Could you check a few things on this model? Use its own coordinates, in mm. Give positions to 0.01 mm unless a question says otherwise; leave off trailing zeros. Loops run counter-clockwise (first coordinate to the right, second up) from the corner with the lowest first, then second, coordinate; pieces in that order, holes last. Notation, with made-up numbers: (76, 57.5) -> (129, 57.5) arc R17 ccw to (129, 63.5) -> close; hole circle Ø2 at (87.25, 49). An arc over 180 degrees is marked (long way). Write each question's results on one line, items separated by ' | '. Start each with the question number.
Q1. If we section it at D-D, the plane x = -46: List the corners of the cut face in (y, z) for me.
Q2. Will these pins go through, and if not, where does the flat tip stop? P1, Ø2, axis at y = 2, z = -66, coming from the +X side; P2, Ø1.2, axis at x = -13.5, y = 3, coming from the +Z side; P3, Ø1, axis at y = 4.5, z = -125, coming from the -X side.
Q3. If I drill on line 1 along Z through (x, y) = (2.5, 1.25); line 2 along Z through (x, y) = (-41, 1.5); line 3 along X through (y, z) = (0.75, -17.5), over which ranges is the centre line in solid material (lowest first)?
Q4. If we section it at C-C, the plane z = -110.5: List the corners of the cut face in (x, y) for me, plus the area to 3 significant figures.
Q5. If we section it at A-A, the plane x = -60: List the corners of the cut face in (y, z) for me, plus the area to 3 significant figures.
Q6. If we section it at B-B, the plane y = 5: Give the number of separate pieces and of enclosed holes in the cut face, plus the area to 3 significant figures.
Autodesk Inventor part; units mm, degrees
ref_plane "YZ Plane" through (0, 0, 0) normal (1, 0, 0) x (0, 1, 0)
ref_plane "XZ Plane" through (0, 0, 0) normal (0, 1, 0) x (-1, 0, 0)
ref_plane "XY Plane" through (0, 0, 0) normal (0, 0, 1) x (1, 0, 0)
sketch "Sketch1" plane through (0, 0, 0) normal (0, 1, 0) x (-1, 0, 0)
  line L0 (8, 0) -> (76.1537, -12.0173)
  line L1 (76.1537, -12.0173) -> (76.1537, -54.5039)
  line L2 (76.1537, -54.5039) -> (9.2866, -150)
  line L3 (0, -150) -> (0, 0)
  line L4 (75.1537, -50.7018) -> (69.8292, -46.9735) construction
  line L5 (69.8292, -46.9735) -> (1, -145.2718) construction
  line L6 (1, -145.2718) -> (6.3245, -149) construction
  line L7 (6.3245, -149) -> (75.1537, -50.7018) construction
  line L8 (75.1537, -14.8873) -> (74.0249, -21.2885) construction
  line L9 (74.0249, -21.2885) -> (1, -8.4123) construction
  line L10 (1, -8.4123) -> (2.1287, -2.011) construction
  line L11 (2.1287, -2.011) -> (75.1537, -14.8873) construction
  line L12 (73.1537, -45.9735) -> (66.6537, -45.9735) construction
  line L13 (66.6537, -45.9735) -> (66.6537, -22.2885) construction
  line L14 (66.6537, -22.2885) -> (73.1537, -22.2885) construction
  line L15 (73.1537, -22.2885) -> (73.1537, -45.9735) construction
  line L16 (0, -150) -> (9.2866, -150)
  line L17 (0, 0) -> (8, 0)
  line L18 (66.6537, -51.5086) -> (66.6537, -19.9888)
  point P0 (0, 0)
  dimension "d0" = 6.5
  dimension "d1" = 3
  dimension "d2" = 3
  dimension "d3" = 3
  dimension "d4" = 120
  dimension "d5" = 80
  dimension "d6" = 35
  dimension "d7" = 1
  dimension "d8" = 1
  dimension "d9" = 1
  dimension "d10" = 1
  dimension "d12" = 1
  dimension "d13" = 8
  dimension "d14" = 150
extrude "Extrusion1" add sketch "Sketch1" along normal blind 6.5
chamfer "Chamfer1" distance 2 angle 45 3 edges at (-76.1537, 3.25, -54.5039) (-76.1537, 3.25, -12.0173) (-9.2866, 3.25, -150)
sketch "Sketch3" plane through (0, 6.5, 0) normal (0, 1, 0) x (1, 0, 0)
  line L0 (-10.4338, 148.3617) -> (-75.0065, 56.1423)
  line L1 (-76.1537, 52.5039) -> (-76.1537, 14.0173)
  line L2 (-74.184, 11.67) -> (-8, 0)
  line L3 (0, 0) -> (0, 150)
  line L4 (0, 150) -> (-7.2866, 150)
  line L5 (-6.3245, 149) -> (-1, 145.2718) construction
  line L6 (-1, 145.2718) -> (-69.8292, 46.9735) construction
  line L7 (-69.8292, 46.9735) -> (-75.1537, 50.7018) construction
  line L8 (-75.1537, 50.7018) -> (-6.3245, 149) construction
  line L9 (-73.1537, 45.9735) -> (-66.6537, 45.9735) construction
  line L10 (-66.6537, 45.9735) -> (-66.6537, 22.2885) construction
  line L11 (-66.6537, 22.2885) -> (-73.1537, 22.2885) construction
  line L12 (-73.1537, 22.2885) -> (-73.1537, 45.9735) construction
  line L13 (-74.0249, 21.2885) -> (-75.1537, 14.8873) construction
  line L14 (-75.1537, 14.8873) -> (-2.1287, 2.011) construction
  line L15 (-2.1287, 2.011) -> (-1, 8.4123) construction
  line L16 (-1, 8.4123) -> (-74.0249, 21.2885) construction
  circle A0 centre (-69.9037, 34.131) radius 2.25
  line L17 (-56.0633, 66.6332) -> (-51.4747, 73.1864)
  line L18 (-51.4747, 73.1864) -> (-56.7992, 76.9146)
  line L19 (-56.7992, 76.9146) -> (-61.3878, 70.3614)
  line L20 (-61.3878, 70.3614) -> (-56.0633, 66.6332)
  line L21 (-37.7089, 92.846) -> (-33.1203, 99.3992)
  line L22 (-33.1203, 99.3992) -> (-38.4448, 103.1275)
  line L23 (-38.4448, 103.1275) -> (-43.0334, 96.5743)
  line L24 (-43.0334, 96.5743) -> (-37.7089, 92.846)
  line L25 (-19.3544, 119.0589) -> (-14.7658, 125.6121)
  line L26 (-14.7658, 125.6121) -> (-20.0903, 129.3404)
  line L27 (-20.0903, 129.3404) -> (-24.6789, 122.7871)
  line L28 (-24.6789, 122.7871) -> (-19.3544, 119.0589)
  line L29 (-72.4914, 48.8376) -> (-58.7256, 68.4973) construction
  line L30 (-54.137, 75.0505) -> (-40.3711, 94.7101) construction
  line L31 (-35.7825, 101.2634) -> (-22.0167, 120.923) construction
  line L32 (-17.4281, 127.4762) -> (-3.6622, 147.1359) construction
  line L33 (-16.3, 112.5) -> (-16.3, 108)
  line L34 (0, 108) -> (0, 112.5)
  line L35 (-12.3, 115) -> (-5, 115)
  line L36 (-5, 105.5) -> (-12.3, 105.5)
  line L37 (0, 112.5) -> (-5, 112.5)
  line L38 (-12.3, 112.5) -> (-16.3, 112.5)
  line L39 (-16.3, 108) -> (-12.3, 108)
  line L40 (-5, 108) -> (0, 108)
  line L41 (-12.3, 105.5) -> (-12.3, 108)
  line L42 (-12.3, 112.5) -> (-12.3, 115)
  line L43 (-5, 115) -> (-5, 112.5)
  line L44 (-5, 108) -> (-5, 105.5)
  line L45 (-70.0857, 20.5939) -> (-62.2073, 19.2048)
  line L46 (-62.2073, 19.2048) -> (-63.336, 12.8035)
  line L47 (-63.336, 12.8035) -> (-71.2144, 14.1927)
  line L48 (-71.2144, 14.1927) -> (-70.0857, 20.5939)
  line L49 (-41.4517, 15.545) -> (-33.5732, 14.1558)
  line L50 (-33.5732, 14.1558) -> (-34.702, 7.7546)
  line L51 (-34.702, 7.7546) -> (-42.5804, 9.1437)
  line L52 (-42.5804, 9.1437) -> (-41.4517, 15.545)
  line L53 (-12.8177, 10.496) -> (-4.9392, 9.1069)
  line L54 (-4.9392, 9.1069) -> (-6.0679, 2.7056)
  line L55 (-6.0679, 2.7056) -> (-13.9464, 4.0948)
  line L56 (-13.9464, 4.0948) -> (-12.8177, 10.496)
  line L57 (-62.7716, 16.0041) -> (-42.0161, 12.3444) construction
  line L58 (-34.1376, 10.9552) -> (-13.382, 7.2954) construction
  circle A1 centre (-52.3938, 14.1742) radius 2.25
  circle A2 centre (-23.7598, 9.1253) radius 2.25
  line L59 (-16.3, 67.975) -> (-16.3, 63.475)
  line L60 (0, 63.475) -> (0, 67.975)
  line L61 (-12.3, 70.475) -> (-5, 70.475)
  line L62 (-5, 60.975) -> (-12.3, 60.975)
  line L63 (0, 67.975) -> (-5, 67.975)
  line L64 (-12.3, 67.975) -> (-16.3, 67.975)
  line L65 (-16.3, 63.475) -> (-12.3, 63.475)
  line L66 (-5, 63.475) -> (0, 63.475)
  line L67 (-12.3, 60.975) -> (-12.3, 63.475)
  line L68 (-12.3, 67.975) -> (-12.3, 70.475)
  line L69 (-5, 70.475) -> (-5, 67.975)
  line L70 (-5, 63.475) -> (-5, 60.975)
  line L71 (-16.3, 23.45) -> (-16.3, 18.95)
  line L72 (0, 18.95) -> (0, 23.45)
  line L73 (-12.3, 25.95) -> (-5, 25.95)
  line L74 (-5, 16.45) -> (-12.3, 16.45)
  line L75 (0, 23.45) -> (-5, 23.45)
  line L76 (-12.3, 23.45) -> (-16.3, 23.45)
  line L77 (-16.3, 18.95) -> (-12.3, 18.95)
  line L78 (-5, 18.95) -> (0, 18.95)
  line L79 (-12.3, 16.45) -> (-12.3, 18.95)
  line L80 (-12.3, 23.45) -> (-12.3, 25.95)
  line L81 (-5, 25.95) -> (-5, 23.45)
  line L82 (-5, 18.95) -> (-5, 16.45)
  line L83 (-8.65, 105.5) -> (-8.65, 70.475) construction
  line L84 (-8.65, 60.975) -> (-8.65, 25.95) construction
  line L85 (-8, 0) -> (0, 0)
  point P0 (-69.9037, 45.9735)
  point P1 (-73.1537, 34.131)
  point P2 (-16.3, 21.2)
  dimension "d25" = 6.5
  dimension "d26" = 3
  dimension "d27" = 3
  dimension "d28" = 3
  dimension "d29" = 120
  dimension "d30" = 1
  dimension "d31" = 1
  dimension "d32" = 1
  dimension "d33" = 1
  dimension "d34" = 1
  dimension "d35" = 4.5
  dimension "d36" = 8
  dimension "d37" = 4.5
  dimension "d38" = 5
  dimension "d39" = 4
  dimension "d40" = 7.3
  dimension "d41" = 2.5
  dimension "d42" = 4
  dimension "d43" = 4
  dimension "d44" = 4.5
  dimension "d45" = 5
  dimension "d46" = 4
  dimension "d47" = 7.3
  dimension "d48" = 2.5
  dimension "d49" = 4.5
  dimension "d50" = 5
  dimension "d51" = 4
  dimension "d52" = 7.3
  dimension "d53" = 2.5
  dimension "d55" = 35
  dimension "d67" = 21.2
extrude "Extrusion3" cut sketch "Sketch3" against normal through all
sketch "Sketch4" plane through (0, 6.5, 0) normal (0, 1, 0) x (1, 0, 0)
  line L0 (0, 67.975) -> (0, 108)
  line L1 (0, 112.5) -> (0, 150)
  line L2 (0, 0) -> (0, 18.95)
  line L3 (-16.3, 18.95) -> (-16.3, 23.45)
  line L4 (0, 23.45) -> (0, 63.475)
  line L5 (0, 135.25) -> (4.5, 135.25)
  line L6 (6.5, 133.25) -> (6.5, 129.25)
  line L7 (4.5, 127.25) -> (0, 127.25)
  line L8 (0, 127.25) -> (0, 135.25)
  line L9 (0, 91.9875) -> (4.5, 91.9875)
  line L10 (6.5, 89.9875) -> (6.5, 85.9875)
  line L11 (4.5, 83.9875) -> (0, 83.9875)
  line L12 (0, 83.9875) -> (0, 91.9875)
  line L13 (0, 47.4625) -> (4.5, 47.4625)
  line L14 (6.5, 45.4625) -> (6.5, 41.4625)
  line L15 (4.5, 39.4625) -> (0, 39.4625)
  line L16 (0, 39.4625) -> (0, 47.4625)
  line L17 (0, 13.7) -> (4.5, 13.7)
  line L18 (6.5, 11.7) -> (6.5, 7.7)
  line L19 (4.5, 5.7) -> (0, 5.7)
  line L20 (0, 5.7) -> (0, 13.7)
  arc A0 (6.5, 133.25) -> (4.5, 135.25) centre (4.5, 133.25) ccw
  arc A1 (4.5, 127.25) -> (6.5, 129.25) centre (4.5, 129.25) ccw
  arc A2 (6.5, 89.9875) -> (4.5, 91.9875) centre (4.5, 89.9875) ccw
  arc A3 (4.5, 83.9875) -> (6.5, 85.9875) centre (4.5, 85.9875) ccw
  arc A4 (6.5, 45.4625) -> (4.5, 47.4625) centre (4.5, 45.4625) ccw
  arc A5 (4.5, 39.4625) -> (6.5, 41.4625) centre (4.5, 41.4625) ccw
  arc A6 (6.5, 11.7) -> (4.5, 13.7) centre (4.5, 11.7) ccw
  arc A7 (4.5, 5.7) -> (6.5, 7.7) centre (4.5, 7.7) ccw
  point P0 (-16.3, 21.2)
  point P1 (6.5, 131.25)
  point P2 (0, 131.25)
  point P3 (6.5, 87.9875)
  point P4 (0, 87.9875)
  point P5 (6.5, 43.4625)
  point P6 (0, 43.4625)
  dimension "d58" = 2
  dimension "d59" = 8
  dimension "d60" = 8
  dimension "d61" = 8
  dimension "d62" = 8
  dimension "d63" = 6.5
  dimension "d64" = 7.5
extrude "Extrusion4" add sketch "Sketch4" against normal blind 6.5
equation "\"d60\" = d59"
equation "\"d61\" = d60"
equation "\"d62\" = d61"
properties part number "front_panel_brace_right" material "Plywood, Finish"
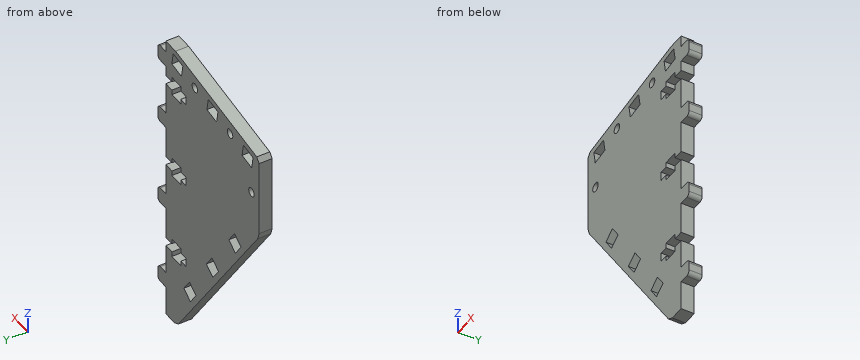
Final values:
1) outline: (0, -97.57) -> (6.5, -97.57) -> (6.5, -6.7) -> (0, -6.7) -> close
2) P1: stops at x = -16.3 | P2: stops at z = -0.86 | P3: stops at x = -27.14
3) line 1: z = -135.25 to -127.25, -91.99 to -83.99, -47.46 to -39.46, -13.7 to -5.7 | line 2: z = -104.71 to -99.48, -95.15 to -15.47, -8.87 to -5.82 | line 3: x = -76.15 to -70.63, -62.51 to -12.3, -5 to 0
4) outline: (-36.94, 0) -> (-16.3, 0) -> (-16.3, 6.5) -> (-36.94, 6.5) -> close | area: 134 mm²
5) outline: (0, -77.57) -> (6.5, -77.57) -> (6.5, -72.34) -> (0, -72.34) -> close; (0, -69.39) -> (6.5, -69.39) -> (6.5, -9.17) -> (0, -9.17) -> close | area: 425 mm²
6) separate pieces: 1 | enclosed holes: 9 | area: 7,330 mm²
